Design review of the part built by this model. Coordinates are the model's own, in mm. Face numbers are marked on the shaded views. Round coordinates to 2 decimals unless told otherwise and drop trailing zeros. Loops run counter-clockwise (first coordinate to the right, second up) from the corner with the lowest first, then second, coordinate; pieces in that order, holes last. Notation, with made-up numbers: (60.25, -36) - (91.25, -36) arc R17 ccw to (91.25, -9) - close; hole circle Ø1 at (56, -29). An arc over 180 degrees is marked (long way). One line per question, with ' | ' between items. Start each with the question number.
from build123d import *

# Parameters (mm, degrees)
F0_R     = 11.2
F1_DEPTH = 1.5
F2_R     = 6
F3_DEPTH = 0.6
F4_R     = 4.05
F5_DEPTH = 3
F6_T     = -1.2
F7_R     = 1.49999
F8_SIZE  = 0.4


# Not quite as in the source:
# - a fillet or chamfer is up to 0.001 mm smaller than in the source, because OpenCascade refuses the exact size


with BuildPart() as f1:
    # F0 (on Top) → F1 (new body)
    with BuildSketch(Plane.XY):
        Circle(F0_R)
    extrude(amount=-F1_DEPTH)

    # F2 (on face) → F3 (join)
    with BuildSketch(Plane.XY):
        Circle(F2_R)
    extrude(amount=F3_DEPTH)

    # F4 (on face) → F5 (join)
    with BuildSketch(Plane.XY.offset(0.6)):
        Circle(F4_R)
    extrude(amount=F5_DEPTH)

    # F6
    f6_openings = [f1.faces().sort_by_distance(p)[0] for p in [
        (0, 0, 3.6),
    ]]
    offset(amount=F6_T, openings=f6_openings, kind=Kind.INTERSECTION)

    # F7 (radius 1.5 in the source; OpenCascade refuses exactly that, so slightly less here)
    f7_edges = [f1.edges().sort_by_distance(p)[0] for p in [
        (-11.2, 0, -1.5),
    ]]
    fillet(f7_edges, radius=F7_R)

    # F8
    f8_edges = [f1.edges().sort_by_distance(p)[0] for p in [
        (-2.85, 0, 3.6),
        (2.85, 0, 1.65),
    ]]
    chamfer(f8_edges, length=F8_SIZE)


solid = f1.part
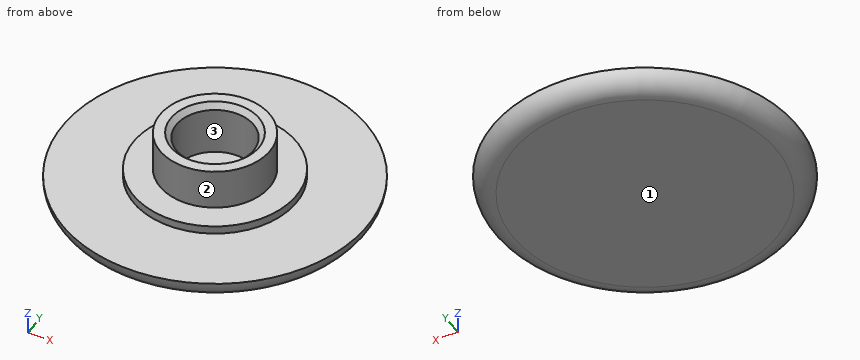
1. The part is to be moulded in two halves that separate along Y. For the marked faces 1, 2 and 3, say which applies: pulls with the +Y half, pulls with the -Y half, needs draft (parallel to the pull), parting line crosses it, or undercut.
2. To check wall thickness, follow line 1 along Y through (x, z) = (0, 1.7); line 2 along Y through (x, z) = (-1.5, -0.2); line 3 along Z through (x, y) = (4.5, -1.25). State the ranges of each line that lie inside material, in increasing order.
3. Take a section at D-D, the plane z = -1. Give the boundary of the cut face in (x, y).
4. Clearance check with flat-ended pins moving along their axes: P1, Ø8, axis at x = 6.5, y = 9, coming from the +Z side; P2, Ø6.5, axis at x = 1.5, y = -0.5, coming from the +Z side; P3, Ø3, axis at y = -4.5, z = -0.5, coming from the +X side; P4, Ø3, axis at x = -2.5, z = 2.5, coming from the -Y side. State where each tip first meets the part, or that it passes through.
5. Take a section at B-B, the plane z = 1.6. Give the boundary of the cut face in (x, y), then the cut area to 3 significant figures.
Answer list:
1) face 1: needs draft | face 2: parting line crosses it | face 3: undercut
2) line 1: y = -4.05 to -2.85, 2.85 to 4.05 | line 2: y = -11.09 to -2.42, 2.42 to 11.09 | line 3: z = -1.5 to 0.6
3) outline: circle Ø21.64 at (0, 0)
4) P1: stops at z = 0 | P2: stops at z = 3.6 | P3: stops at x = 10.77 | P4: stops at y = -3.92
5) outline: circle Ø8.1 at (0, 0); hole circle Ø5.7 at (0, 0) | area: 26.0 mm²
